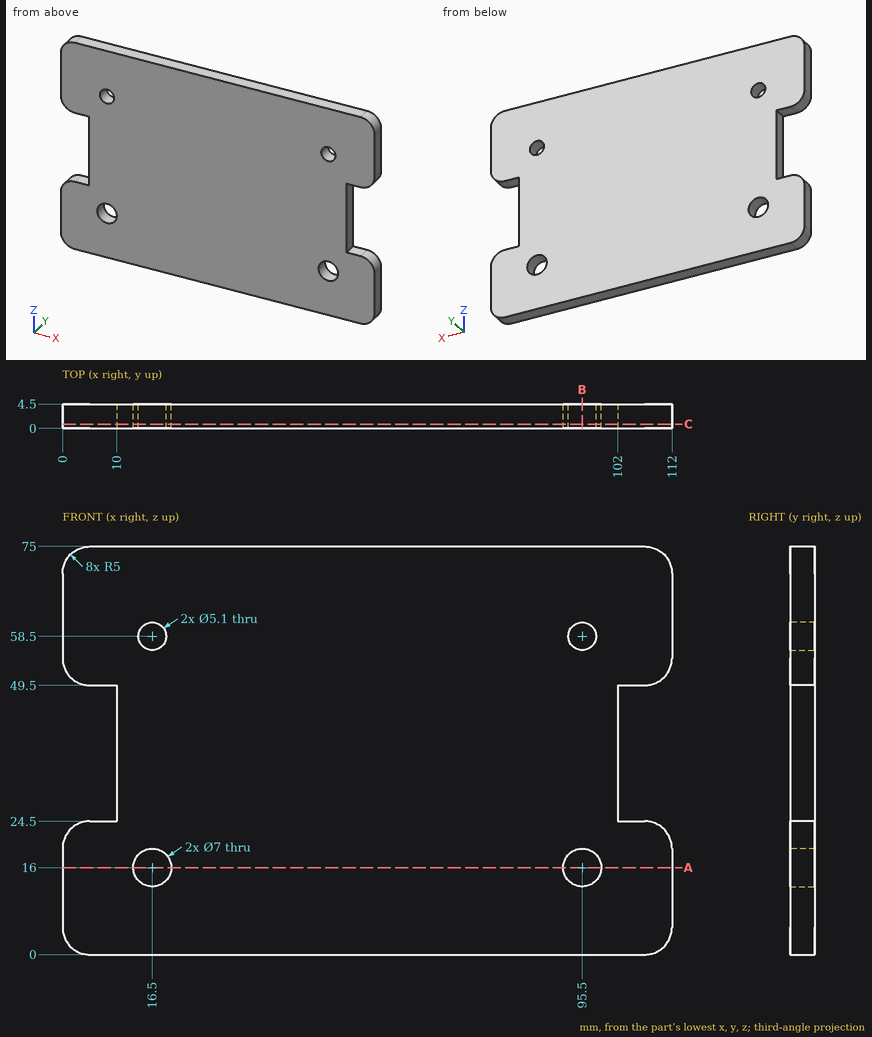
The drawing under review shows one solid part. Ordinate dimensions are in mm from its lowest x, y, z. Coordinates: 2 decimals unless noted, no trailing zeros. Loops run counter-clockwise (first coordinate to the right, second up) from the corner with the lowest first, then second, coordinate; pieces in that order, holes last. Notation, with made-up numbers: (68.25, 23) - (126.25, 23) arc R11 cw to (126.25, 42) - close; hole circle Ø3 at (63.25, 10.5). An arc over 180 degrees is marked (long way). Use CSV: the item, a comma, the result in double quotes. Start each with the question number.
1. Clearance check with flat-ended pins moving along their axes: pin 1 (2 mm diameter, centred on y = 3.5, z = 21.5, fed in from -X); pin 2 (1.3 mm diameter, centred on y = 2.5, z = 34, fed in from -X); pin 3 (1.3 mm diameter, centred on y = 1.5, z = 33.5, fed in from +X). State where each tip first meets the part, or that it passes through.
2. Add section A-A on z = 16. Give the boundary of the cut face in (x, y).
3. Add section C-C on y = 0.8. Give the boundary of the cut face in (x, z).
4. To check wall thickness, follow probe 1 along X at (y, z) = (1.55, 58.5); probe 2 along X at (y, z) = (0.95, 16); probe 3 along Z at (x, y) = (17.5, 3.75). State the ranges of each line that lie inside material, in increasing order.
5. Add section B-B on x = 95.5. Give the boundary of the cut face in (y, z), plus the area to 3 significant figures.
Resolved:
1,pin 1,"x = 0.1"
1,pin 2,"x = 10"
1,pin 3,"x = 102"
2,outline,"(0, 0) - (13, 0) - (13, 4.5) - (0, 4.5) - close; (20, 0) - (92, 0) - (92, 4.5) - (20, 4.5) - close; (99, 0) - (112, 0) - (112, 4.5) - (99, 4.5) - close"
3,outline,"(0, 5) arc R5 ccw to (5, 0) - (107, 0) arc R5 ccw to (112, 5) - (112, 19.5) arc R5 ccw to (107, 24.5) - (102, 24.5) - (102, 49.5) - (107, 49.5) arc R5 ccw to (112, 54.5) - (112, 70) arc R5 ccw to (107, 75) - (5, 75) arc R5 ccw to (0, 70) - (0, 54.5) arc R5 ccw to (5, 49.5) - (10, 49.5) - (10, 24.5) - (5, 24.5) arc R5 ccw to (0, 19.5) - close; hole circle Ø7 at (16.5, 16); hole circle Ø5.1 at (16.5, 58.5); hole circle Ø7 at (95.5, 16); hole circle Ø5.1 at (95.5, 58.5)"
4,probe 1,"0 to 13.95, 19.05 to 92.95, 98.05 to 112"
4,probe 2,"0 to 13, 20 to 92, 99 to 112"
4,probe 3,"0 to 12.65, 19.35 to 56.15, 60.85 to 75"
5,outline,"(0, 0) - (4.5, 0) - (4.5, 12.5) - (0, 12.5) - close; (0, 19.5) - (4.5, 19.5) - (4.5, 55.95) - (0, 55.95) - close; (0, 61.05) - (4.5, 61.05) - (4.5, 75) - (0, 75) - close"
5,area,"283 mm2"
